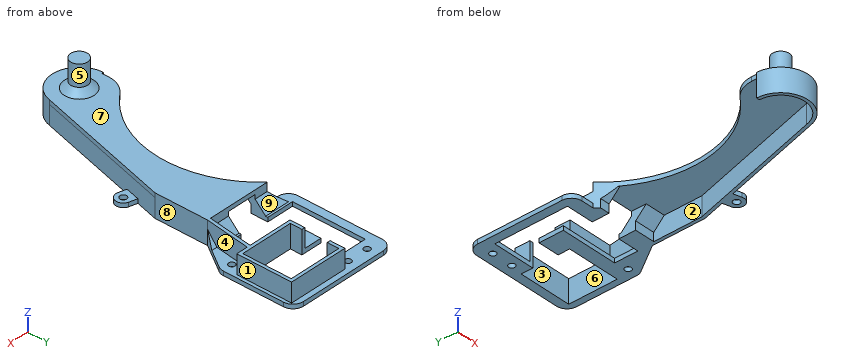
from build123d import *

# Parameters (mm, degrees)
EXTRUDE_1_DEPTH                 = 52
CUT_EXTRUDE_1_REACH             = 161.013
CUT_EXTRUDE_1_DIRECTION_2_DEPTH = 7
SKETCH_3_R                      = 1.5
CUT_EXTRUDE_2_DEPTH             = 160.138304628
SKETCH_5_R                      = 4
EXTRUDE_3_DEPTH                 = 15
FILLET_1_R                      = 5
CHAMFER_1_SIZE                  = 5
FILLET_2_R                      = 12.5
EXTRUDE_2_DEPTH                 = 9
CHAMFER_2_SIZE                  = 5
EXTRUDE_4_DEPTH                 = 9
EXTRUDE_4_DEPTH_BACK            = 2
CHAMFER_3_SIZE                  = 3
SKETCH_7_R                      = 1.6
EXTRUDE_5_DEPTH                 = 2


with BuildPart() as part:
    # 草图1 → 凸台-拉伸1 (new body)
    with BuildSketch(Plane(origin=(0, 0, 0), x_dir=(0, 0, -1), z_dir=(1, 0, 0))):
        Polygon((0, 0), (0, 98), (9, 98), (9, 150), (7, 150), (7, 100), (-2, 100), (-2, 0), align=None)
    extrude(amount=EXTRUDE_1_DEPTH)

    # 草图2 → 切除-拉伸1 (cut, up to next)
    with BuildSketch(Plane.XY.offset(-7), mode=Mode.PRIVATE) as cut_extrude_1_sk1:
        Polygon((24, 146), (49, 146), (49, 123), (24, 123), (24, 128.5), (14, 128.5), (14, 117), (41, 117), (41, 106), (31, 106), (31, 98), (17, 98), (17, 106), (4, 106), (4, 140.5), (24, 140.5), align=None)
    cut_extrude_1_tool1 = extrude(cut_extrude_1_sk1.sketch, amount=-CUT_EXTRUDE_1_REACH, mode=Mode.PRIVATE) & part.part
    add(cut_extrude_1_tool1.solids().sort_by_distance((25.692202, 124.595066, -7))[0], mode=Mode.SUBTRACT)

    # 草图2 → 切除-拉伸1 direction 2 (cut)
    with BuildSketch(Plane.XY.offset(-7)):
        Polygon((24, 146), (49, 146), (49, 123), (24, 123), (24, 128.5), (14, 128.5), (14, 117), (41, 117), (41, 106), (31, 106), (31, 98), (17, 98), (17, 106), (4, 106), (4, 140.5), (24, 140.5), align=None)
    extrude(amount=CUT_EXTRUDE_1_DIRECTION_2_DEPTH, mode=Mode.SUBTRACT)

    # 草图3 → 切除-拉伸2 (cut, through all)
    with BuildSketch(Plane.XY.offset(2)):
        with Locations((8, 145)):
            Circle(SKETCH_3_R)
        with Locations((18, 145)):
            Circle(SKETCH_3_R)
        with Locations((47, 116)):
            Circle(SKETCH_3_R)
        with BuildLine():
            Line((0, 100), (10.707142143, 100))
            ThreePointArc((10.707142143, 100), (24.538989746, 58.225895269), (0, 21.698729811))
            Line((0, 21.698729811), (0, 100))
        make_face()
        Polygon((42, 75), (42, 100), (52, 115), (52, 0), (22, 0), align=None)
    extrude(amount=-CUT_EXTRUDE_2_DEPTH, mode=Mode.SUBTRACT)

    # 草图5 → 凸台-拉伸3 (add)
    with BuildSketch(Plane(origin=(0, 0, 0), x_dir=(-1, 0, 0), z_dir=(0, 0, -1))):
        with Locations(Location((-12, 12, 0), (0, 0, 90))):
            Circle(SKETCH_5_R)
    extrude(amount=-EXTRUDE_3_DEPTH)

    # 圆角1
    fillet_1_edges = [part.edges().sort_by_distance(p)[0] for p in [
        (52, 115, -8),
        (0, 100, -8),
        (52, 150, -8),
        (0, 150, -8),
    ]]
    fillet(fillet_1_edges, radius=FILLET_1_R)

    # 倒角1
    chamfer_1_edges = [part.edges().sort_by_distance(p)[0] for p in [
        (13.853571071, 100, -7),
        (36.5, 100, -7),
    ]]
    chamfer(chamfer_1_edges, length=CHAMFER_1_SIZE)

    # 圆角2
    # the kernel refuses this fillet: 12.5 mm, written as the material it takes off along each edge
    with BuildSketch(Plane(origin=(0, 0, 33.25), x_dir=(1, 0, 0), z_dir=(0, 0, -1))) as fillet_2_piece_1:
        with BuildLine():
            CenterArc((FILLET_2_R, -FILLET_2_R), FILLET_2_R, 90, 90)
            Line((0, -FILLET_2_R), (0, 0))
            Line((0, 0), (FILLET_2_R, 0))
        make_face()
    extrude(amount=64.5, mode=Mode.SUBTRACT)
    with BuildSketch(Plane(origin=(22, 0, 26.008697284), x_dir=(0.2576626505603325, 0.9662349396012462, 0), z_dir=(0, 0, -1))) as fillet_2_piece_2:
        with BuildLine():
            CenterArc((FILLET_2_R * 0.768278313084, -FILLET_2_R), FILLET_2_R, 90, 75.068582822)
            Line((-FILLET_2_R * 0.197956626517, -FILLET_2_R * 0.74233734944), (0, 0))
            Line((0, 0), (FILLET_2_R * 0.768278313084, 0))
        make_face()
    extrude(amount=50.017394568, mode=Mode.SUBTRACT)
    with BuildSketch(Plane(origin=(0, 21.698729811, 18.746824527), x_dir=(0.8345119301206998, 0.550989871491504, 0), z_dir=(0, 0, -1))) as fillet_2_piece_3:
        with BuildLine():
            CenterArc((6.740466849, 12.477543337), FILLET_2_R, 213.434948823, 53.130102354)
            Line((-3.690932278, 5.590169944), (0, 0))
            ThreePointArc((0, 0), (2.995763044, 0.08982665), (5.991526088, 0))
        make_face()
    extrude(amount=35.493649054, mode=Mode.SUBTRACT)

    # 草图4 → 凸台-拉伸2 (add)
    with BuildSketch(Plane.XY.offset(-7)):
        Polygon((24, 128.5), (24, 123), (49, 123), (49, 146), (24, 146), (24, 140.5), (22.5, 140.5), (22.5, 147.5), (50.5, 147.5), (50.5, 121.5), (45, 121.5), (42, 100), (40.485467906, 100), (43.485467906, 121.5), (22.5, 121.5), (22.5, 128.5), align=None)
    extrude(amount=EXTRUDE_2_DEPTH)

    # 倒角2
    chamfer_2_edges = [part.edges().sort_by_distance(p)[0] for p in [
        (14.781639971, 98, 0),
        (36.5, 98, 0),
    ]]
    chamfer(chamfer_2_edges, length=CHAMFER_2_SIZE)

    # 草图6 → 凸台-拉伸4 (add, two sides: drawn at the far end of the back side and taken through both)
    with BuildSketch(Plane(origin=(0, 0, 0), x_dir=(-1, 0, 0), z_dir=(0, 0, -1)).offset(-EXTRUDE_4_DEPTH_BACK)):
        with BuildLine():
            Line((-40.5, 100), (-42, 100))
            Line((-42, 100), (-42, 75))
            Line((-42, 75), (-24.474457831, 9.279216868))
            ThreePointArc((-24.474457831, 9.279216868), (-10.631728691, -0.694195235), (0.76772333, 12))
            Line((0.76772333, 12), (-0.727521137, 12))
            ThreePointArc((-0.727521137, 12), (-10.853296347, 0.785997572), (-23.03917982, 9.718489836))
            Line((-23.03917982, 9.718489836), (-40.5, 75.196565511))
            Line((-40.5, 75.196565511), (-40.5, 100))
        make_face()
    extrude(amount=EXTRUDE_4_DEPTH + EXTRUDE_4_DEPTH_BACK)

    # 倒角3
    chamfer_3_edges = [part.edges().sort_by_distance(p)[0] for p in [
        (12, 8, 2),
    ]]
    chamfer(chamfer_3_edges, length=CHAMFER_3_SIZE)

    # 草图7 → 凸台-拉伸5 (add)
    with BuildSketch(Plane(origin=(0, 0, -9), x_dir=(-1, 0, 0), z_dir=(0, 0, -1))):
        with BuildLine():
            Line((-39.167379443, 64.377672911), (-42.901819277, 63.381822289))
            ThreePointArc((-42.901819277, 63.381822289), (-45.381822289, 59.098180723), (-41.098180723, 56.618177711))
            Line((-41.098180723, 56.618177711), (-37.363740889, 57.614028334))
            Line((-37.363740889, 57.614028334), (-39.167379443, 64.377672911))
        make_face()
        with Locations(Location((-42, 60, 0), (0, 0, 90))):
            Circle(SKETCH_7_R, mode=Mode.SUBTRACT)
    extrude(amount=-EXTRUDE_5_DEPTH)


solid = part.part
Read the model definition and answer for the solid it produces. Units are mm, in the model's axes. Face numbers are marked on the shaded views. A direction names the side the tool comes from. Give positions to 0.01 mm unless a question says otherwise; leave off trailing zeros. Write each loop counter-clockwise with the first axis right and the second up, starting at its lowest first coordinate (ties: lowest second). Pieces come first, ordered by that corner, then holes. Notation, with made-up numbers: (-20, -10.75) - (34, -10.75) arc R26 cw to (34, 10.25) - close; hole circle Ø8 at (25, 49). An arc over 180 degrees is marked (long way). Use CSV: the item, a comma, the result in double quotes. Start each with the question number.
(1) Find section A-A (y = 136). Give the vertices of the cut face in (x, z).
(2) For the marked faces 1, 2, 3, 4 and 5, determine the directions among +Z, -Z, +X, -X, +Y, -Y from which every point of the face is accessible in a straight line to the end or side of a thin tool.
(3) Find section C-C (z = 9.5). Give the vertices of the cut face in (x, y).
(4) Given P1, Ø3, axis at x = 27, y = 87, coming from the -Z side; P2, Ø12, axis at x = 16.5, z = -2, coming from the -Y side; P3, Ø3, axis at y = 78.5, z = -1.5, coming from the +X side; P4, Ø5.5, axis at y = 125, z = -4.5, coming from the -X side, each flat-ended and moving along its own axis, determine where each tip first touches the part or whether it passes through.
(5) Find section D-D (y = 96). Give the vertices of the cut face in (x, z).
(6) Determine the mould class of the marked faces 6, 7, 8 and 9 for opening direction Y: +Y half, -Y half, draft (parallel to the pull), parting line (faces both ways), or undercut.
(7) Consider line 1 along X through (y, z) = (145, -8.35); line 2 along X through (y, z) = (116, -8.25); line 3 along Y through (x, z) = (8, -8.15). Determine where each line is inside the solid, lowest interval first.
(8) Find section B-B (y = 45.5). Give the vertices of the cut face in (x, z).
Findings below:
1,outline,"(0, -9) - (4, -9) - (4, -7) - (0, -7) - close; (49, -9) - (52, -9) - (52, -7) - (50.5, -7) - (50.5, 2) - (49, 2) - close"
2,face 1,"+Z, +X, +Y, -Y"
2,face 2,"-Z, -X"
2,face 3,"+Z, -Z"
2,face 4,"+Z, +X"
2,face 5,"+Z"
3,outline,"circle Ø8 at (12, 12)"
4,P1,"z = 0"
4,P2,"y = -0.77"
4,P3,"x = 42"
4,P4,"x = 0"
5,outline,"(14.23, -3) - (17, -3) - (17, 0) - (31, 0) - (31, -3) - (40.5, -3) - (40.5, -9) - (42, -9) - (42, 2) - (14.23, 2) - close"
6,face 6,"undercut"
6,face 7,"draft"
6,face 8,"undercut"
6,face 9,"+Y half"
7,line 1,"0 to 6.5, 9.5 to 16.5, 19.5 to 24, 49 to 52"
7,line 2,"0 to 4, 41 to 45.5, 48.5 to 51.97"
7,line 3,"-0.12 to 1.46, 100 to 106, 140.5 to 143.5, 146.5 to 150"
8,outline,"(21.04, 0) - (32.58, 0) - (32.58, -9) - (34.13, -9) - (34.13, 2) - (21.04, 2) - close"
